Verification items for the finished model (mm, model axes). Face numbers are marked on the shaded views. Give positions to 0.01 mm unless a question says otherwise; leave off trailing zeros. Write each loop counter-clockwise with the first axis right and the second up, starting at its lowest first coordinate (ties: lowest second). Pieces come first, ordered by that corner, then holes. Notation, with made-up numbers: (40.25, 26.25) -> (56.25, 26.25) arc R35 ccw to (56.25, 58.25) -> close; hole circle Ø1 at (5, -24.75). An arc over 180 degrees is marked (long way). Answer as CSV lines item,"result". Start each with the question number.
1) Gauge pin test, flat ends, axial feed: pin 1 Ø6 at (x, y) = (3, 8) entering from -Z; pin 2 Ø3 at (y, z) = (-3, 6) entering from -X; pin 3 Ø3 at (x, y) = (6.5, 8) entering from +Z; pin 4 Ø4 at (x, z) = (-8, 8.5) entering from -Y. Record the tip position at first contact, or that the pin passes through.
2) Sectioned sample at A-A on y = 0. Record the cut outline in (x, z), and give its area (3 significant figures).
3) Mould release check, pull along Y, two halves, no side actions. Record for the marked faces 1, 2, 3 and 4: released by +Y, released by -Y, zero draft, split by the parting line, or undercut.
4) Material ranges on L1, parallel to Y at x = 0, z = 4.75; L2, parallel to Y at x = 10, z = 7.5; L3, parallel to Z at x = 6.75, y = -9.75, recorded low to high.
```python
from build123d import *

# Parameters (mm, degrees)
F0_R     = 8.35
F0_R_2   = 6.35
F1_DEPTH = 12
F2_DEPTH = 10
F3_R     = 1


with BuildPart() as f1:
    # F0 (on Top) → F1 (new body)
    with BuildSketch(Plane.XY):
        Circle(F0_R)
        Circle(F0_R_2, mode=Mode.SUBTRACT)
    extrude(amount=F1_DEPTH)

    # F0 (on Top) → F2 (join)
    with BuildSketch(Plane.XY):
        with BuildLine():
            ThreePointArc((12.925266, 0.4), (13.216714, 0.526033), (13.324502, 0.82471))
            ThreePointArc((13.324502, 0.82471), (13.185639, 2.0884), (12.927204, 3.333151))
            ThreePointArc((12.927204, 3.333151), (12.732395, 3.583902), (12.416265, 3.613704))
            Line((12.416265, 3.613704), (12.059366, 3.497741))
            Line((12.059366, 3.497741), (11.812152, 4.258586))
            Line((11.812152, 4.258586), (12.169052, 4.374549))
            ThreePointArc((12.169052, 4.374549), (12.407289, 4.584476), (12.417505, 4.901844))
            ThreePointArc((12.417505, 4.901844), (11.894937, 6.060773), (11.264501, 7.164741))
            ThreePointArc((11.264501, 7.164741), (11.001741, 7.34302), (10.691874, 7.273674))
            Line((10.691874, 7.273674), (10.388277, 7.053098))
            Line((10.388277, 7.053098), (9.918049, 7.700312))
            Line((9.918049, 7.700312), (10.221646, 7.920888))
            ThreePointArc((10.221646, 7.920888), (10.383352, 8.194159), (10.294996, 8.499151))
            ThreePointArc((10.294996, 8.499151), (9.439876, 9.439876), (8.499151, 10.294996))
            ThreePointArc((8.499151, 10.294996), (8.194159, 10.383352), (7.920888, 10.221646))
            Line((7.920888, 10.221646), (7.700312, 9.918049))
            Line((7.700312, 9.918049), (7.053098, 10.388277))
            Line((7.053098, 10.388277), (7.273674, 10.691874))
            ThreePointArc((7.273674, 10.691874), (7.34302, 11.001741), (7.164741, 11.264501))
            ThreePointArc((7.164741, 11.264501), (6.060773, 11.894937), (4.901844, 12.417505))
            ThreePointArc((4.901844, 12.417505), (4.584476, 12.407289), (4.374549, 12.169052))
            Line((4.374549, 12.169052), (4.258586, 11.812152))
            Line((4.258586, 11.812152), (3.497741, 12.059366))
            Line((3.497741, 12.059366), (3.613704, 12.416265))
            ThreePointArc((3.613704, 12.416265), (3.583902, 12.732395), (3.333151, 12.927204))
            ThreePointArc((3.333151, 12.927204), (2.0884, 13.185639), (0.82471, 13.324502))
            ThreePointArc((0.82471, 13.324502), (0.526033, 13.216714), (0.4, 12.925266))
            Line((0.4, 12.925266), (0.4, 12.55))
            Line((0.4, 12.55), (-0.4, 12.55))
            Line((-0.4, 12.55), (-0.4, 12.925266))
            ThreePointArc((-0.4, 12.925266), (-0.526033, 13.216714), (-0.82471, 13.324502))
            ThreePointArc((-0.82471, 13.324502), (-2.0884, 13.185639), (-3.333151, 12.927204))
            ThreePointArc((-3.333151, 12.927204), (-3.583902, 12.732395), (-3.613704, 12.416265))
            Line((-3.613704, 12.416265), (-3.497741, 12.059366))
            Line((-3.497741, 12.059366), (-4.258586, 11.812152))
            Line((-4.258586, 11.812152), (-4.374549, 12.169052))
            ThreePointArc((-4.374549, 12.169052), (-4.584476, 12.407289), (-4.901844, 12.417505))
            ThreePointArc((-4.901844, 12.417505), (-6.060773, 11.894937), (-7.164741, 11.264501))
            ThreePointArc((-7.164741, 11.264501), (-7.34302, 11.001741), (-7.273674, 10.691874))
            Line((-7.273674, 10.691874), (-7.053098, 10.388277))
            Line((-7.053098, 10.388277), (-7.700312, 9.918049))
            Line((-7.700312, 9.918049), (-7.920888, 10.221646))
            ThreePointArc((-7.920888, 10.221646), (-8.194159, 10.383352), (-8.499151, 10.294996))
            ThreePointArc((-8.499151, 10.294996), (-9.439876, 9.439876), (-10.294996, 8.499151))
            ThreePointArc((-10.294996, 8.499151), (-10.383352, 8.194159), (-10.221646, 7.920888))
            Line((-10.221646, 7.920888), (-9.918049, 7.700312))
            Line((-9.918049, 7.700312), (-10.388277, 7.053098))
            Line((-10.388277, 7.053098), (-10.691874, 7.273674))
            ThreePointArc((-10.691874, 7.273674), (-11.001741, 7.34302), (-11.264501, 7.164741))
            ThreePointArc((-11.264501, 7.164741), (-11.894937, 6.060773), (-12.417505, 4.901844))
            ThreePointArc((-12.417505, 4.901844), (-12.407289, 4.584476), (-12.169052, 4.374549))
            Line((-12.169052, 4.374549), (-11.812152, 4.258586))
            Line((-11.812152, 4.258586), (-12.059366, 3.497741))
            Line((-12.059366, 3.497741), (-12.416265, 3.613704))
            ThreePointArc((-12.416265, 3.613704), (-12.732395, 3.583902), (-12.927204, 3.333151))
            ThreePointArc((-12.927204, 3.333151), (-13.185639, 2.0884), (-13.324502, 0.82471))
            ThreePointArc((-13.324502, 0.82471), (-13.216714, 0.526033), (-12.925266, 0.4))
            Line((-12.925266, 0.4), (-12.55, 0.4))
            Line((-12.55, 0.4), (-12.55, -0.4))
            Line((-12.55, -0.4), (-12.925266, -0.4))
            ThreePointArc((-12.925266, -0.4), (-13.216714, -0.526033), (-13.324502, -0.82471))
            ThreePointArc((-13.324502, -0.82471), (-13.185639, -2.0884), (-12.927204, -3.333151))
            ThreePointArc((-12.927204, -3.333151), (-12.732395, -3.583902), (-12.416265, -3.613704))
            Line((-12.416265, -3.613704), (-12.059366, -3.497741))
            Line((-12.059366, -3.497741), (-11.812152, -4.258586))
            Line((-11.812152, -4.258586), (-12.169052, -4.374549))
            ThreePointArc((-12.169052, -4.374549), (-12.407289, -4.584476), (-12.417505, -4.901844))
            ThreePointArc((-12.417505, -4.901844), (-11.894937, -6.060773), (-11.264501, -7.164741))
            ThreePointArc((-11.264501, -7.164741), (-11.001741, -7.34302), (-10.691874, -7.273674))
            Line((-10.691874, -7.273674), (-10.388277, -7.053098))
            Line((-10.388277, -7.053098), (-9.918049, -7.700312))
            Line((-9.918049, -7.700312), (-10.221646, -7.920888))
            ThreePointArc((-10.221646, -7.920888), (-10.383352, -8.194159), (-10.294996, -8.499151))
            ThreePointArc((-10.294996, -8.499151), (-9.439876, -9.439876), (-8.499151, -10.294996))
            ThreePointArc((-8.499151, -10.294996), (-8.194159, -10.383352), (-7.920888, -10.221646))
            Line((-7.920888, -10.221646), (-7.700312, -9.918049))
            Line((-7.700312, -9.918049), (-7.053098, -10.388277))
            Line((-7.053098, -10.388277), (-7.273674, -10.691874))
            ThreePointArc((-7.273674, -10.691874), (-7.34302, -11.001741), (-7.164741, -11.264501))
            ThreePointArc((-7.164741, -11.264501), (-6.060773, -11.894937), (-4.901844, -12.417505))
            ThreePointArc((-4.901844, -12.417505), (-4.584476, -12.407289), (-4.374549, -12.169052))
            Line((-4.374549, -12.169052), (-4.258586, -11.812152))
            Line((-4.258586, -11.812152), (-3.497741, -12.059366))
            Line((-3.497741, -12.059366), (-3.613704, -12.416265))
            ThreePointArc((-3.613704, -12.416265), (-3.583902, -12.732395), (-3.333151, -12.927204))
            ThreePointArc((-3.333151, -12.927204), (-2.0884, -13.185639), (-0.82471, -13.324502))
            ThreePointArc((-0.82471, -13.324502), (-0.526033, -13.216714), (-0.4, -12.925266))
            Line((-0.4, -12.925266), (-0.4, -12.55))
            Line((-0.4, -12.55), (0.4, -12.55))
            Line((0.4, -12.55), (0.4, -12.925266))
            ThreePointArc((0.4, -12.925266), (0.526033, -13.216714), (0.82471, -13.324502))
            ThreePointArc((0.82471, -13.324502), (2.0884, -13.185639), (3.333151, -12.927204))
            ThreePointArc((3.333151, -12.927204), (3.583902, -12.732395), (3.613704, -12.416265))
            Line((3.613704, -12.416265), (3.497741, -12.059366))
            Line((3.497741, -12.059366), (4.258586, -11.812152))
            Line((4.258586, -11.812152), (4.374549, -12.169052))
            ThreePointArc((4.374549, -12.169052), (4.584476, -12.407289), (4.901844, -12.417505))
            ThreePointArc((4.901844, -12.417505), (6.060773, -11.894937), (7.164741, -11.264501))
            ThreePointArc((7.164741, -11.264501), (7.34302, -11.001741), (7.273674, -10.691874))
            Line((7.273674, -10.691874), (7.053098, -10.388277))
            Line((7.053098, -10.388277), (7.700312, -9.918049))
            Line((7.700312, -9.918049), (7.920888, -10.221646))
            ThreePointArc((7.920888, -10.221646), (8.194159, -10.383352), (8.499151, -10.294996))
            ThreePointArc((8.499151, -10.294996), (9.439876, -9.439876), (10.294996, -8.499151))
            ThreePointArc((10.294996, -8.499151), (10.383352, -8.194159), (10.221646, -7.920888))
            Line((10.221646, -7.920888), (9.918049, -7.700312))
            Line((9.918049, -7.700312), (10.388277, -7.053098))
            Line((10.388277, -7.053098), (10.691874, -7.273674))
            ThreePointArc((10.691874, -7.273674), (11.001741, -7.34302), (11.264501, -7.164741))
            ThreePointArc((11.264501, -7.164741), (11.894937, -6.060773), (12.417505, -4.901844))
            ThreePointArc((12.417505, -4.901844), (12.407289, -4.584476), (12.169052, -4.374549))
            Line((12.169052, -4.374549), (11.812152, -4.258586))
            Line((11.812152, -4.258586), (12.059366, -3.497741))
            Line((12.059366, -3.497741), (12.416265, -3.613704))
            ThreePointArc((12.416265, -3.613704), (12.732395, -3.583902), (12.927204, -3.333151))
            ThreePointArc((12.927204, -3.333151), (13.185639, -2.0884), (13.324502, -0.82471))
            ThreePointArc((13.324502, -0.82471), (13.216714, -0.526033), (12.925266, -0.4))
            Line((12.925266, -0.4), (12.55, -0.4))
            Line((12.55, -0.4), (12.55, 0.4))
            Line((12.55, 0.4), (12.925266, 0.4))
        make_face()
        Circle(F0_R, mode=Mode.SUBTRACT)
    extrude(amount=F2_DEPTH)

    # F3
    f3_edges = [f1.edges().sort_by_distance(p)[0] for p in [
        (-6.35, 0, 12),
    ]]
    fillet(f3_edges, radius=F3_R)


solid = f1.part
```
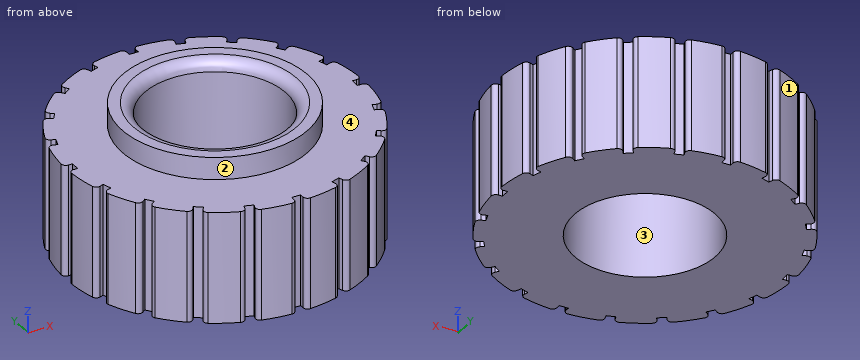
Ans:
1,pin 1,"stops at z = 0"
1,pin 2,"stops at x = -13.27"
1,pin 3,"stops at z = 10"
1,pin 4,"stops at y = -11.93"
2,outline,"(-12.55, 0) -> (-6.35, 0) -> (-6.35, 11) arc R1 ccw to (-7.35, 12) -> (-8.35, 12) -> (-8.35, 10) -> (-12.55, 10) -> close; (6.35, 0) -> (12.55, 0) -> (12.55, 10) -> (8.35, 10) -> (8.35, 12) -> (7.35, 12) arc R1 ccw to (6.35, 11) -> close"
2,area,"132 mm²"
3,face 1,"released by +Y"
3,face 2,"split by the parting line"
3,face 3,"undercut"
3,face 4,"zero draft"
4,L1,"y = -12.55 to -6.35, 6.35 to 12.55"
4,L2,"y = -8.84 to -7.76, -7.59 to 7.59, 7.76 to 8.84"
4,L3,"z = 0 to 10"
